Geometry: final body of the model. Coordinates: model frame, mm. Coordinates: 2 decimals unless noted, no trailing zeros. Write each loop counter-clockwise with the first axis right and the second up, starting at its lowest first coordinate (ties: lowest second). Pieces come first, ordered by that corner, then holes. Notation, with made-up numbers: (13, 66.5) - (57, 66.5) arc R36 ccw to (57, 105.5) - close; hole circle Ø8 at (73.5, 30.5). An arc over 180 degrees is marked (long way). Answer as a JSON object with one key per item and string values. Group by question number.
Item 1: First-contact query: pin 1 Ø6 at (y, z) = (-59, 97.5) entering from +X; pin 2 Ø12 at (x, z) = (-59.5, 99) entering from -Y; pin 3 Ø2 at (x, z) = (0.5, 1.5) entering from -Y. Flat tips, straight axial feed; report the tip coordinate or a pass-through.
Item 2: Line query: line 1 along X through (y, z) = (-49, 86.5); line 2 along Z through (x, y) = (-58, -57). Output: solid intervals per line, ascending. Write a range as from..to.
Item 3: Section A-A on x = -14.5. Return loops of the section in (y, z), and give its area (3 significant figures).
Item 4: Section B-B on z = 78. Return loops of the section in (x, y).
Autodesk Inventor part; units mm, degrees
ref_plane "Arbeitsebene1" through (0, 0, 3) normal (-0.7071068, 0.7071068, 0) x (0.7071068, 0.7071068, 0)
ref_plane "Arbeitsebene2" through (0, 0, 3) normal (0, 0.8564105, 0.5162955) x (-0.4587597, -0.4587597, 0.7609724)
ref_plane "YZ Plane" through (0, 0, 0) normal (1, 0, 0) x (0, 1, 0)
sketch "Skizze1" plane through (0, 0, 0) normal (0, 0, 1) x (1, 0, 0)
  line L0 (0, 0) -> (2, 0)
  line L1 (2, 0) -> (2, 2)
  line L2 (2, 2) -> (0, 2)
  line L3 (0, 2) -> (0, 0)
  dimension "d0" = 2
  dimension "d1" = 2
extrude "Extrusion1" add sketch "Skizze1" along normal blind 3
sketch "Skizze2" plane through (0, 0, 3) normal (0, 0, 1) x (1, 0, 0)
  point P0 (0, 0)
ref_plane "Arbeitsebene1" through (0, 0, 3) normal (-0.7071068, 0.7071068, 0) x (0.7071068, 0.7071068, 0)
sketch "Skizze3" plane through (0, 0, 3) normal (-0.7071068, 0.7071068, 0) x (0.7071068, 0.7071068, 0)
  line L0 (0, 0) -> (1.4142, 0)
  line L1 (0, 0) -> (-112.5245, -131.9823)
  line L2 (0, 0) -> (173.439, 0) construction
  line L3 (2.8284, 3) -> (2.8284, 0)
  line L4 (2.8284, 0) -> (-109.6961, -131.9823)
  line L5 (2.8284, 0) -> (176.2674, 0) construction
  line L6 (-109.6961, -131.9823) -> (-112.5245, -131.9823)
  line L7 (1.4142, 0) -> (2.8284, 0)
  line L8 (2.8284, 0) -> (0, 0)
  point P0 (0, 3)
  dimension "d4" = 173.439
  dimension "d5" = 130.45
  dimension "d6" = 173.439
  dimension "d7" = 130.45
ref_plane "Arbeitsebene2" through (0, 0, 3) normal (0, 0.8564105, 0.5162955) x (-0.4587597, -0.4587597, 0.7609724)
sketch "Skizze4" plane through (0, 0, 3) normal (0, 0.8564105, 0.5162955) x (-0.4587597, -0.4587597, 0.7609724)
  line L0 (0, 0) -> (-0.9175, 1.7771)
  line L1 (0, 0) -> (-0.9175, 1.7771)
  line L2 (-0.9175, 1.7771) -> (172.5215, 1.7771)
  line L3 (172.5215, 1.7771) -> (173.439, 0)
  line L4 (173.439, 0) -> (0, 0)
  point P0 (-2.2829, -1.1787)
  dimension "d9" = 173.439
extrude "Extrusion2" add sketch "Skizze4" along normal blind 2
sketch "Skizze5" plane through (-77.5668, -79.5668, 134.9823) normal (0.8885604, -0.2368556, 0.3928866) x (0.4587597, 0.4587597, -0.7609724)
  line L0 (172.5215, 0) -> (-0.9175, 0)
  line L1 (0.0005, 0) -> (1.3553, 2)
  line L2 (0, 2) -> (173.439, 2)
  line L3 (1.3553, 2) -> (0, 2)
  line L4 (0, 0) -> (0, 2)
  line L5 (0, 2) -> (0, 0)
  point P0 (174.8044, -1.5489)
sketch "Skizze6" plane through (0, 0, 3) normal (0, -0.8564105, -0.5162955) x (0.8885604, -0.2368556, 0.3928866)
  line L0 (0, 0) -> (0, 173.439)
  line L1 (1.7771, 172.5215) -> (0, 173.439)
  point P0 (-1.1787, -2.2829)
sketch "Skizze7" plane through (0, 1.7128, 4.0326) normal (0, 0.8564105, 0.5162955) x (0.8885604, -0.2368556, 0.3928866)
  line L0 (0, 0) -> (0, -173.439)
  line L1 (0, -172.1027) -> (1.781, -171.1647)
  point P0 (-1.1787, 2.2829)
sketch "Skizze8" plane through (0, 0, 3) normal (-0.8885604, 0.2368556, -0.3928866) x (-0.4587597, -0.4587597, 0.7609724)
  line L0 (0, 2) -> (173.439, 2)
  line L1 (0, 0) -> (173.439, 0)
  line L2 (172.1026, 2) -> (173.439, 0)
  point P0 (-2.2829, -1.5489)
chamfer "Fase1" distance 1.1929 distance2 2 1 edges at (-78.5668, -77.854, 136.0149) measured on face at (-25.1889, -24.8095, 48.0267)
ref_plane "Arbeitsebene3" through (2, 0, 3) normal (-1, 0, 0) x (0, 0.8564105, 0.5162955)
sketch "Skizze12" plane through (2, 0, 3) normal (-1, 0, 0) x (0, 0.8564105, 0.5162955)
  line L0 (0, 0) -> (1.7128, 1.0326)
  line L1 (0, 0) -> (2, 0)
  line L2 (-1.5489, 2.5692) -> (0, 0)
  line L3 (0, 0) -> (1.7128, 1.0326)
  line L4 (2, 0) -> (1.7128, 1.0326)
extrude "Extrusion6" add sketch "Skizze12" along normal blind 2
sketch "Skizze13" plane through (0, 0, 0) normal (0, 0, -1) x (-1, 0, 0)
  line L0 (0, 2) -> (0, 0)
  line L1 (-2, 0) -> (-2, 2)
  line L2 (0, 0) -> (-2, 0)
  line L3 (-2, 0) -> (-2, 2)
  line L4 (-2, 2) -> (0, 2)
  line L5 (0, 2) -> (0, 0)
extrude "Extrusion7" add sketch "Skizze13" along normal blind 2
properties part number "FOVStick"
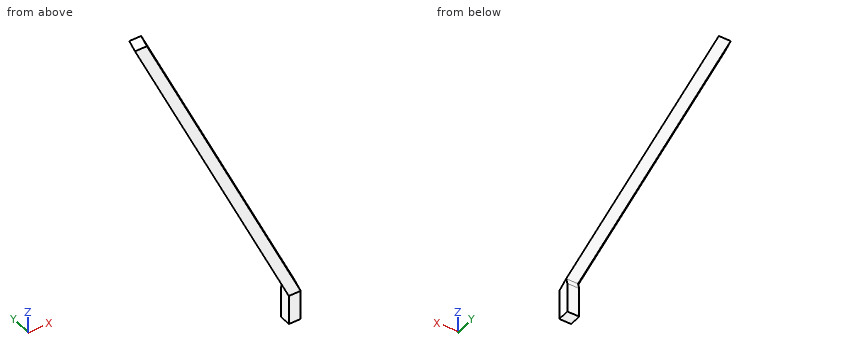
Checks:
{
 "1": {"pin 1": "x = -54.25", "pin 2": "y = -61.49", "pin 3": "y = 0"},
 "2": {"line 1": "-49.98..-47.98", "line 2": "99.81..101.42"},
 "3": {"outline": "(-16.5, 30.37) - (-14.5, 27.05) - (-12.79, 28.08) - (-14.79, 31.4) - close", "area": "7.75 mm^2"},
 "4": {"outline": "(-45.21, -45.21) - (-43.21, -45.21) - (-42.59, -42.88) - (-44.59, -42.88) - close"}
}
